Design review of the part built by this model. Coordinates are the model's own, in mm. Face numbers are marked on the shaded views. A direction names the side the tool comes from. Give positions to 0.01 mm unless a question says otherwise; leave off trailing zeros. Loops run counter-clockwise (first coordinate to the right, second up) from the corner with the lowest first, then second, coordinate; pieces in that order, holes last. Notation, with made-up numbers: (-19.75, 14) - (-4.75, 14) arc R22 cw to (-4.75, 50) - close; hole circle Ø5 at (14, 4.25). An arc over 180 degrees is marked (long way). Write each question's results on one line, items separated by ' | '.
from build123d import *

# Parameters (mm, degrees)
F0_W          = 127
F0_H          = 190.5
F1_DEPTH      = 9.525
F3_DEPTH      = 76.2
F3_DEPTH_BACK = 38.1
F4_DEPTH      = 38.1
F4_DEPTH_BACK = 76.2
F6_DEPTH      = 88.9


with BuildPart() as f1:
    # F0 (on Front) → F1 (new body, symmetric)
    with BuildSketch(Plane.XZ):
        Rectangle(F0_W, F0_H)
    extrude(amount=F1_DEPTH, both=True)

    # F2 (on Top) → F3 (join, two sides)
    with BuildSketch(Plane.XY) as f3_sk:
        with BuildLine():
            Line((-38.1, -9.525), (-44.45, -9.525))
            Line((-44.45, -9.525), (-44.45, -28.575))
            ThreePointArc((-44.45, -28.575), (-49.0985226281, -62.0897721088), (-19.05, -46.5355122421))
            Line((-19.05, -46.5355122421), (-24.638, -46.5355122421))
            ThreePointArc((-24.638, -46.5355122421), (-47.6190714883, -56.0545837305), (-38.1, -33.0735122421))
            Line((-38.1, -33.0735122421), (-38.1, -9.525))
        make_face()
        with BuildLine():
            Line((-31.75, -9.525), (-38.1, -9.525))
            Line((-38.1, -9.525), (-38.1, -33.0735122421))
            ThreePointArc((-38.1, -33.0735122421), (-28.5809285117, -37.0164407538), (-24.638, -46.5355122421))
            Line((-24.638, -46.5355122421), (-19.05, -46.5355122421))
            ThreePointArc((-19.05, -46.5355122421), (-22.5457401333, -35.5369896141), (-31.75, -28.575))
            Line((-31.75, -28.575), (-31.75, -9.525))
        make_face()
    extrude(amount=F3_DEPTH)
    extrude(f3_sk.sketch, amount=-F3_DEPTH_BACK)

    # F2 (on Top) → F4 (join, two sides)
    with BuildSketch(Plane.XY) as f4_sk:
        with BuildLine():
            Line((24.638, -46.5355122421), (19.05, -46.5355122421))
            ThreePointArc((19.05, -46.5355122421), (49.0985226281, -62.0897721088), (44.45, -28.575))
            Line((44.45, -28.575), (44.45, -9.525))
            Line((44.45, -9.525), (38.1, -9.525))
            Line((38.1, -9.525), (38.1, -33.0735122421))
            ThreePointArc((38.1, -33.0735122421), (47.6190714883, -37.0164407538), (51.562, -46.5355122421))
            ThreePointArc((51.562, -46.5355122421), (38.1, -59.9975122421), (24.638, -46.5355122421))
        make_face()
        with BuildLine():
            ThreePointArc((31.75, -28.575), (22.5457401333, -35.5369896141), (19.05, -46.5355122421))
            Line((19.05, -46.5355122421), (24.638, -46.5355122421))
            ThreePointArc((24.638, -46.5355122421), (28.5809285117, -37.0164407538), (38.1, -33.0735122421))
            Line((38.1, -33.0735122421), (38.1, -9.525))
            Line((38.1, -9.525), (31.75, -9.525))
            Line((31.75, -9.525), (31.75, -28.575))
        make_face()
    extrude(amount=F4_DEPTH)
    extrude(f4_sk.sketch, amount=-F4_DEPTH_BACK)

    # F5 (on Top) → F6 (join, symmetric)
    with BuildSketch(Plane.XY):
        with BuildLine():
            Line((-7.9375, 27.5268467149), (-7.9375, 9.525))
            Line((-7.9375, 9.525), (0, 9.525))
            Line((0, 9.525), (7.9375, 9.525))
            Line((7.9375, 9.525), (7.9375, 27.5268467149))
            ThreePointArc((7.9375, 27.5268467149), (0, 25.4), (-7.9375, 27.5268467149))
        make_face()
        with BuildLine():
            ThreePointArc((15.875, 41.275), (-7.9375, 55.0231532851), (-7.9375, 27.5268467149))
            ThreePointArc((-7.9375, 27.5268467149), (0, 25.4), (7.9375, 27.5268467149))
            ThreePointArc((7.9375, 27.5268467149), (13.7481532851, 33.3375), (15.875, 41.275))
        make_face()
    extrude(amount=F6_DEPTH, both=True)


solid = f1.part
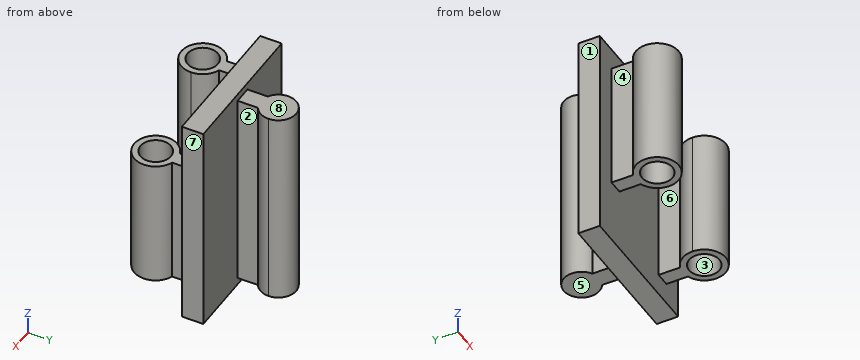
(1) Draft analysis for pull direction X (two halves, no side actions). For the marked faces 6, 7 and 8, state which applies: pulls with the +X half, pulls with the -X half, needs draft (parallel to the pull), parting line crosses it, or undercut.
Answers below:
face 6: undercut | face 7: pulls with the +X half | face 8: needs draft
(2) Take a section at D-D on z = -26.5. Count the separate pieces of the cut face and the enclosed holes in it, plus the area to 3 significant figures.
Answers below:
separate pieces: 1 | enclosed holes: 2 | area: 5,080 mm2
(3) Tool access review of the marked faces 1, 2, 3, 4 and 5: name each direction out of +Z, -Z, +X, -X, +Y, -Y from which nothing blocks a thin tool from reaching the whole face with its end or side.
Answers below:
face 1: +Z, -Z, -X, +Y, -Y | face 2: +Z, -Z, +X | face 3: +Z, -Z | face 4: +Z, -Z, -X | face 5: -Z, +X, -X, +Y
(4) Wall thickness on line 1 along Y through (x, z) = (29, 30) (3 decimals); line 2 along Y through (x, z) = (-38.1, 19.5) (3 decimals); line 3 along Y through (x, z) = (-49.5, -33.5) (1 decimal): over which ranges is each line inside the solid? List them lowest first. Write a range as from..to.
Answers below:
line 1: -63.271..-56.456, -36.615..-29.8, -9.525..9.525 | line 2: -65.586..-59.998, -33.074..9.525 | line 3: -61.8..-53.7, -39.4..-31.3, -9.5..9.5
(5) Insertion check: P1, Ø9, axis at y = 15.5, z = 18.5, coming from the -X side; P2, Ø12, axis at x = 21.5, z = 9.5, coming from the -Y side; P3, Ø1.5, axis at x = -27, z = -26.5, coming from the +Y side (3 decimals). Each pin has a flat end and moves straight along its axis. Give the tip position at first contact, or say it passes through.
Answers below:
P1: x = -7.94 | P2: y = -62.36 | P3: y = 9.525
(6) Take a section at A-A on x = -38.1. Give the boundary of the cut face in (y, z) (3 decimals), plus the area to 3 significant figures.
Answers below:
outline: (-65.586, -38.1) - (-59.998, -38.1) - (-59.998, 76.2) - (-65.586, 76.2) - close; (-33.074, -38.1) - (-9.525, -38.1) - (-9.525, -95.25) - (9.525, -95.25) - (9.525, 95.25) - (-9.525, 95.25) - (-9.525, 76.2) - (-33.074, 76.2) - close | area: 6,960 mm2
(7) Take a section at B-B on y = -15. Give the boundary of the cut face in (x, z), plus the area to 3 significant figures.
Answers below:
outline: (-44.45, -38.1) - (-31.75, -38.1) - (-31.75, 76.2) - (-44.45, 76.2) - close; (31.75, -76.2) - (44.45, -76.2) - (44.45, 38.1) - (31.75, 38.1) - close | area: 2,900 mm2
